Could you check a few things on this drawing? It's one solid part, dimensions in mm from its lowest x, y, z. Round coordinates to 2 decimals unless told otherwise and drop trailing zeros. Loops run counter-clockwise (first coordinate to the right, second up) from the corner with the lowest first, then second, coordinate; pieces in that order, holes last. Notation, with made-up numbers: M 10,80 L 66,80 A29 cw 66,111 Z; hole C 33,57.5 d6. An arc over 180 degrees is marked long. Answer as CSV lines item,"result".
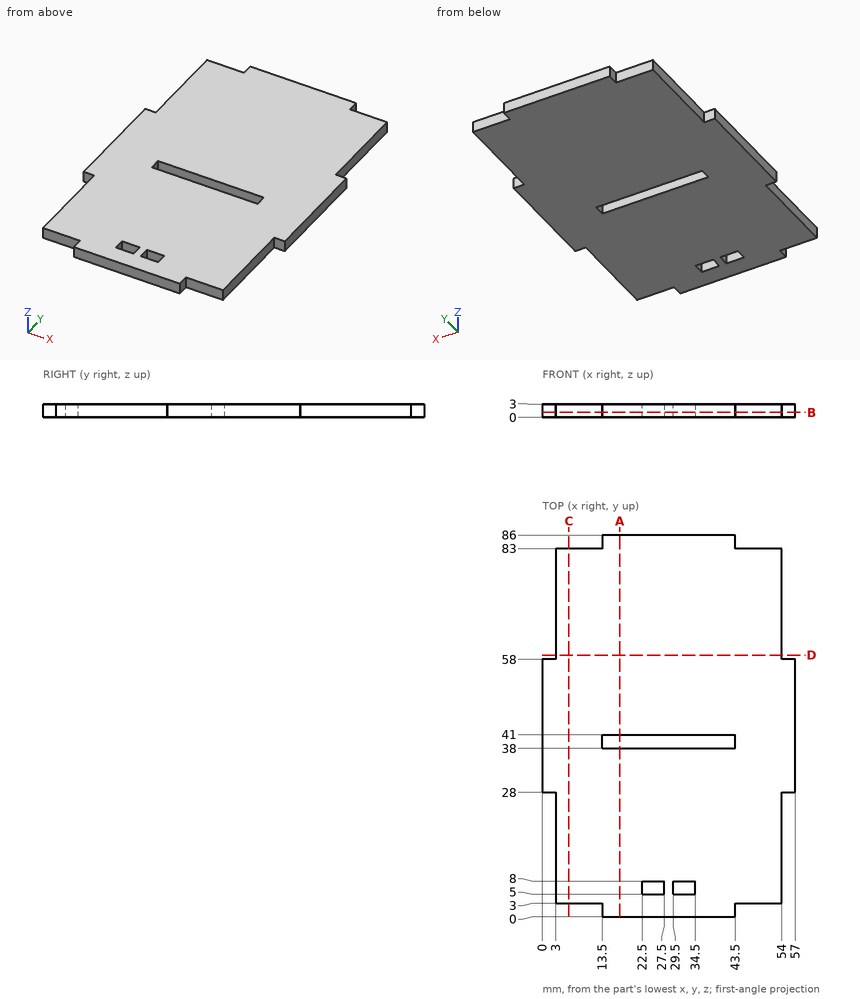
Item 1: If we section it at A-A on x = 17.5: Write out the boundary of the cut face in (y, z), then the cut area to 3 significant figures.
Output:
outline,"M 0,0 L 38,0 L 38,3 L 0,3 Z; M 41,0 L 86,0 L 86,3 L 41,3 Z"
area,"249 mm2"
Item 2: If we section it at B-B on z = 1.1: State how many separate pieces and enclosed holes the cut face has, then the cut area to 3 significant figures.
Output:
separate pieces,"1"
enclosed holes,"3"
area,"4,320 mm2"
Item 3: If we section it at C-C on x = 6: Write out the boundary of the cut face in (y, z), then the cut area to 3 significant figures.
Output:
outline,"M 3,0 L 83,0 L 83,3 L 3,3 Z"
area,"240 mm2"
Item 4: Will these pins go through, and if not, where does the flat tip stop? pin 1 (1.5 mm diameter, centred on x = 56, z = 2, fed in from +Y); pin 2 (1.5 mm diameter, centred on y = 6, z = 2, fed in from -X); pin 3 (12 mm diameter, centred on x = 16.5, y = 75.5, fed in from -Z); pin 4 (1.5 mm diameter, centred on y = 84.5, z = 1, fed in from +X).
Output:
pin 1,"stops at y = 58"
pin 2,"stops at x = 3"
pin 3,"stops at z = 0"
pin 4,"stops at x = 43.5"
Item 5: If I drill on line 1 along Y through (x, z) = (33, 2.25); line 2 along Y through (x, z) = (42, 2.75); line 3 along X through (y, z) = (26.5, 1.2), over which ranges is the centre line in solid material (lowest first)? Write a range as from..to.
Output:
line 1,"y = 0..5, 8..38, 41..86"
line 2,"y = 0..38, 41..86"
line 3,"x = 3..54"
Item 6: If we section it at D-D on y = 59: Write out the boundary of the cut face in (x, z), then the cut area to 3 significant figures.
Output:
outline,"M 3,0 L 54,0 L 54,3 L 3,3 Z"
area,"153 mm2"
